The listing builds one solid part. Answer for the finished solid, in the listing's coordinates (mm). Face numbers are marked on the shaded views. A direction names the side the tool comes from. Give positions to 0.01 mm unless a question says otherwise; leave off trailing zeros. Order: outer loops, then holes, each group sorted by start corner. A loop starts at its lowest first (then second) coordinate and runs counter-clockwise, first axis right, second up. Notation, with made-up numbers: (62, 65) - (85, 65) arc R15 cw to (85, 89) - close; hole circle Ø7 at (-39, -0.5). An arc over 180 degrees is marked (long way). Use CSV: the item, a comma, the result in double quotes.
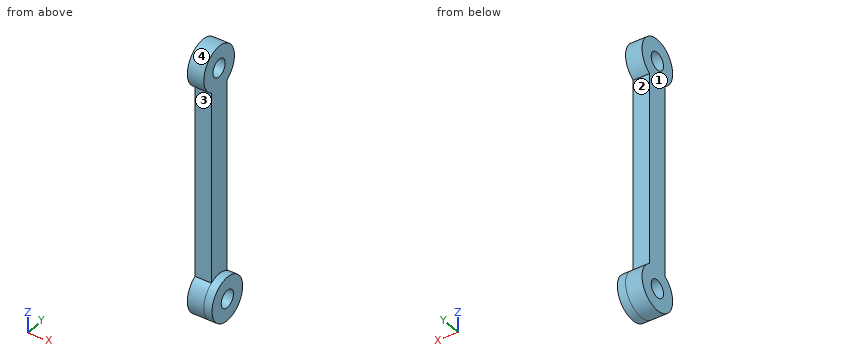
```python
from build123d import *

# Parameters (mm, degrees)
SKETCH1_R           = 1.6
BOSS_EXTRUDE1_DEPTH = 3
SKETCH3_R           = 4
SKETCH3_R_2         = 1.6
BOSS_EXTRUDE3_DEPTH = 1.5


with BuildPart() as part:
    # Sketch1 → Boss-Extrude1 (new body)
    with BuildSketch(Plane(origin=(0, 0, 0), x_dir=(0, 0, -1), z_dir=(1, 0, 0))):
        with BuildLine():
            Line((21, 2), (38.535898385, 2))
            ThreePointArc((38.535898385, 2), (46, 0), (38.535898385, -2))
            Line((38.535898385, -2), (21, -2))
            Line((21, -2), (3.464101615, -2))
            ThreePointArc((3.464101615, -2), (-4, 0), (3.464101615, 2))
            Line((3.464101615, 2), (21, 2))
        make_face()
        Circle(SKETCH1_R, mode=Mode.SUBTRACT)
        with Locations((42, 0)):
            Circle(SKETCH1_R, mode=Mode.SUBTRACT)
    extrude(amount=BOSS_EXTRUDE1_DEPTH)

    # Sketch3 → Boss-Extrude3 (add)
    with BuildSketch(Plane(origin=(3, 0, 0), x_dir=(0, 0, -1), z_dir=(1, 0, 0))):
        with Locations(Location((42, 0, 0), (0, 0, 150))):
            Circle(SKETCH3_R)
        with Locations((42, 0)):
            Circle(SKETCH3_R_2, mode=Mode.SUBTRACT)
    extrude(amount=BOSS_EXTRUDE3_DEPTH)


solid = part.part
```
Item 1: The mould has two halves that part along Z. Classify the marked faces 1 and 2: +Z half, -Z half, draft (parallel to the pull), parting line (faces both ways), or undercut.
Taken from the geometry:
face 1,"draft"
face 2,"undercut"
Item 2: Find the intervals of material crossed by line 1 along Y through (x, z) = (1.75, -42); line 2 along Z through (x, y) = (1.45, -0.75); line 3 along X through (y, z) = (-1, -19.5), in increasing order.
Taken from the geometry:
line 1,"-4 to -1.6, 1.6 to 4"
line 2,"-45.93 to -43.41, -40.59 to -1.41, 1.41 to 3.93"
line 3,"0 to 3"
Item 3: The part is cut by section D-D (z = -42). Give the vertices of the cut face in (x, y).
Taken from the geometry:
outline,"(0, -4) - (4.5, -4) - (4.5, -1.6) - (0, -1.6) - close; (0, 1.6) - (4.5, 1.6) - (4.5, 4) - (0, 4) - close"
Item 4: Which of the six approach directions +Z, -Z, +X, -X, +Y, -Y give full straight-line access (tool end or side, diameter ignored) to the marked faces 3 and 4?
Taken from the geometry:
face 3,"+X, -X, -Y"
face 4,"+X, -X"
Item 5: The part is cut by section A-A (z = 0). Give the vertices of the cut face in (x, y).
Taken from the geometry:
outline,"(0, -4) - (3, -4) - (3, -1.6) - (0, -1.6) - close; (0, 1.6) - (3, 1.6) - (3, 4) - (0, 4) - close"
Item 6: The part is cut by section B-B (y = 0). Give the vertices of the cut face in (x, z).
Taken from the geometry:
outline,"(0, -46) - (4.5, -46) - (4.5, -43.6) - (0, -43.6) - close; (0, -40.4) - (4.5, -40.4) - (4.5, -38) - (3, -38) - (3, -1.6) - (0, -1.6) - close; (0, 1.6) - (3, 1.6) - (3, 4) - (0, 4) - close"
Item 7: The part is cut by section C-C (y = 2.75). Give the vertices of the cut face in (x, z), and give its area (3 significant figures).
Taken from the geometry:
outline,"(0, -44.9) - (4.5, -44.9) - (4.5, -39.1) - (0, -39.1) - close; (0, -2.9) - (3, -2.9) - (3, 2.9) - (0, 2.9) - close"
area,"43.6 mm^2"
Item 8: Each of these flat-tipped pins is pushed along its axis until it touches: pin 1 (2 mm diameter, centred on y = 1.5, z = -28, fed in from -X); pin 2 (2 mm diameter, centred on x = 3.5, y = -3, fed in from +Z); pin 3 (1.5 mm diameter, centred on x = 1.5, z = -25.5, fed in from +Y); pin 4 (1 mm diameter, centred on y = -0.5, z = -21, fed in from +X). Where does it stop, or does it pass through?
Taken from the geometry:
pin 1,"x = 0"
pin 2,"z = 3.38"
pin 3,"y = 2"
pin 4,"x = 3"
